Check sheet for the modelled part. Datum: model origin and axes. Units: mm. A direction names the side the tool comes from. Round coordinates to 2 decimals unless told otherwise and drop trailing zeros. Order: outer loops, then holes, each group sorted by start corner. A loop starts at its lowest first (then second) coordinate and runs counter-clockwise, first axis right, second up.
```python
from build123d import *

# Parameters (mm, degrees)
SKETCH_1_W      = 20
SKETCH_1_H      = 15
SKETCH_1_R      = 1.3
EXTRUDE_1_DEPTH = 1.5
SKETCH_2_W      = 20
SKETCH_2_H      = 4
EXTRUDE_2_DEPTH = 5


with BuildPart() as part:
    # 草图1 → 凸台-拉伸1 (new body)
    with BuildSketch(Plane(origin=(0, 0, 0), x_dir=(1, 0, 0), z_dir=(0, 1, 0))):
        Rectangle(SKETCH_1_W, SKETCH_1_H)
        with Locations(Location((7.5, 0, 0), (0, 0, 270))):
            Circle(SKETCH_1_R, mode=Mode.SUBTRACT)
        with Locations(Location((-7.5, 0, 0), (0, 0, 270))):
            Circle(SKETCH_1_R, mode=Mode.SUBTRACT)
    extrude(amount=EXTRUDE_1_DEPTH)

    # 草图2 → 凸台-拉伸2 (add)
    with BuildSketch(Plane(origin=(0, 1.5, 0), x_dir=(1, 0, 0), z_dir=(0, 1, 0))):
        with Locations((0, 5.5)):
            Rectangle(SKETCH_2_W, SKETCH_2_H)
        with Locations((0, -5.5)):
            Rectangle(SKETCH_2_W, SKETCH_2_H)
    extrude(amount=EXTRUDE_2_DEPTH)


solid = part.part
```
Item 1: Release check for a two-part mould opening along Z. For faces 3 (the flat face through (0, 6.5, -6)), 4 (the flat face through (0, 3, 7.5)), 5 (the flat face through (0, 1.5, 0)) record: released by +Z, released by -Z, zero draft, split by the parting line, or undercut.
Answer:
face 3: zero draft
face 4: released by +Z
face 5: undercut
Item 2: Sectioned sample at A-A (z = 0.5). Record the cut outline in (x, y).
Answer:
outline: (-10, 0) - (-8.7, 0) - (-8.7, 1.5) - (-10, 1.5) - close; (-6.3, 0) - (6.3, 0) - (6.3, 1.5) - (-6.3, 1.5) - close; (8.7, 0) - (10, 0) - (10, 1.5) - (8.7, 1.5) - close
Item 3: Sectioned sample at D-D (x = -0.75). Record the cut outline in (y, z), and give its area (3 significant figures).
Answer:
outline: (0, -7.5) - (6.5, -7.5) - (6.5, -3.5) - (1.5, -3.5) - (1.5, 3.5) - (6.5, 3.5) - (6.5, 7.5) - (0, 7.5) - close
area: 62.5 mm2
Item 4: Go/stop test with a flat-tipped pin: P1, Ø3.5, axis at x = -7.5, z = 0, coming from the +Y side. Record where the tip stops, or that it passes through.
Answer:
P1: stops at y = 1.5
Item 5: Scan lines: line 1 along X through (y, z) = (0.55, 0); line 2 along Z through (x, y) = (3.25, 2); line 3 along Y through (x, z) = (7, 3). Record each from-to range of solid material in increasing order.
Answer:
line 1: x = -10 to -8.8, -6.2 to 6.2, 8.8 to 10
line 2: z = -7.5 to -3.5, 3.5 to 7.5
line 3: y = 0 to 1.5
Item 6: Sectioned sample at C-C (y = 3.75). Record the cut outline in (x, z).
Answer:
outline: (-10, -7.5) - (10, -7.5) - (10, -3.5) - (-10, -3.5) - close; (-10, 3.5) - (10, 3.5) - (10, 7.5) - (-10, 7.5) - close
Item 7: Sectioned sample at B-B (x = -7.5). Record the cut outline in (y, z).
Answer:
outline: (0, -7.5) - (6.5, -7.5) - (6.5, -3.5) - (1.5, -3.5) - (1.5, -1.3) - (0, -1.3) - close; (0, 1.3) - (1.5, 1.3) - (1.5, 3.5) - (6.5, 3.5) - (6.5, 7.5) - (0, 7.5) - close
Item 8: Access from +Z, -Z, +X, -X, +Y, -Y to the whole of each face (thin tool, end or side, straight path). Record for faces 1 (the cylindrical face through (-8.77, 0.74, -0.28)), 2 (the flat face through (0, 4, -3.5)).
Answer:
face 1: +Y, -Y
face 2: +X, -X, +Y
